Verification items for the finished model (mm, model axes). A direction names the side the tool comes from. Round coordinates to 2 decimals unless told otherwise and drop trailing zeros. Order: outer loops, then holes, each group sorted by start corner. A loop starts at its lowest first (then second) coordinate and runs counter-clockwise, first axis right, second up. Notation, with made-up numbers: (53, 17.5) -> (58, 17.5) arc R6 ccw to (58, 22.5) -> close; hole circle Ø2 at (57, 83.25). An arc over 180 degrees is marked (long way). Return JSON: item names as keys, results as strings. Group by question number.
1) Draft check along X on faces 1 (the cylindrical face through (75.86, 5.64, 12.11)), 2 (the flat face through (86, 25, 12)), 3 (the cylindrical face through (0.71, 50.39, 4.7)). Enter one of: pulls with the +X half, pulls with the -X half, needs draft (parallel to the pull), parting line crosses it, or undercut.
2) Tool access check on faces 4 (the flat face through (2.5, 26, 12)), 5 (the cylindrical face through (83.04, 38.95, 13.05)), 6 (the flat face through (4, 0.4, 4)). Record the directions out of +Z, -Z, +X, -X, +Y, -Y that give a thin tool (end or side, any length) a straight path to the whole face; none if there is none.
3) Section check A-A on x = 30. Enter the section's corners in (y, z).
4) Section check B-B on y = 40.6. Enter the section's corners in (x, z), plus the area to 3 significant figures.
5) Section check C-C on z = 10.5. Enter the section's corners in (x, y).
6) Section check D-D on x = 77.25. Enter the section's corners in (y, z).
7) Depth check by flat-ended pin: pin 1 (2.5 mm diameter, centred on x = 77.25, z = 13, fed in from +Y); pin 2 (1 mm diameter, centred on x = 77.5, z = 12.5, fed in from -Y); pin 3 (6 mm diameter, centred on x = 56, z = 13.5, fed in from -Y). Enter the tip coordinate at first touch or a pass-through.
8) Scan lines: L1, parallel to X at y = 5.8, z = 13; L2, parallel to Z at x = 11, y = 4; L3, parallel to X at y = 21, z = 15.75. Record each from-to range of solid material in increasing order.
Autodesk Fusion 360 part; units mm, degrees
sketch "base" plane through (0, 0, 0) normal (0, 0, 1) x (1, 0, 0)
  line L0 (0, 0) -> (88.5, 0)
  line L1 (88.5, 0) -> (88.5, 48.643)
  line L2 (86, 51.143) -> (2.5, 51.143)
  line L3 (0, 48.643) -> (0, 0)
  arc A0 (2.5, 51.143) -> (0, 48.643) centre (2.5, 48.643) ccw
  arc A1 (88.5, 48.643) -> (86, 51.143) centre (86, 48.643) ccw
  point P0 (0, 51.143)
  dimension "d1" = 88.5
  dimension "d2" = 51.143
  dimension "d14" = 2.5
  dimension "d15" = 2.5
extrude "Extrude1" add sketch "base" along normal blind 8
sketch "inside part" plane through (0, 0, 8) normal (0, 0, 1) x (-1, 0, 0)
  line L0 (0, -48.643) -> (0, 0)
  line L1 (0, 0) -> (-88.5, 0)
  line L2 (-88.5, 0) -> (-88.5, -48.643)
  line L3 (-86, -51.143) -> (-2.5, -51.143)
  line L4 (-2.5, 0) -> (-86, 0)
  line L5 (-86, 0) -> (-86, -48.381)
  line L6 (-85.238, -49.143) -> (-3.262, -49.143)
  line L7 (-2.5, -48.381) -> (-2.5, 0)
  arc A0 (-3.262, -49.143) -> (-2.5, -48.381) centre (-3.262, -48.381) ccw
  arc A1 (-86, -48.381) -> (-85.238, -49.143) centre (-85.238, -48.381) ccw
  arc A2 (-88.5, -48.643) -> (-86, -51.143) centre (-86, -48.643) ccw
  arc A3 (-2.5, -51.143) -> (0, -48.643) centre (-2.5, -48.643) ccw
  dimension "d7" = 2.5
  dimension "d8" = 2.5
  dimension "d9" = 2
  dimension "d12" = 0.762
  dimension "d13" = 0.762
extrude "Extrude2" add sketch "inside part" along normal blind 8 contours L1 L4 L5 L6 L7 A0 A1
fillet "Fillet1" radius 1.5 5 edges at (88.5, 24.3215, 0) (87.7678, 50.4108, 0) (44.25, 51.143, 0) (0.7322, 50.4108, 0) (0, 24.3215, 0)
sketch "Sketch3" plane through (0, 0, 0) normal (0, -1, 0) x (1, 0, 0)
  arc A0 (87, 0) -> (88.5, 1.5) centre (87, 1.5) ccw
  line L0 (88.5, 1.5) -> (88.5, 8)
  line L1 (88.5, 8) -> (86, 8)
  line L2 (86, 8) -> (86, 16)
  line L3 (86, 16) -> (2.5, 16)
  line L4 (2.5, 16) -> (2.5, 8)
  line L5 (2.5, 8) -> (0, 8)
  line L6 (0, 8) -> (0, 1.5)
  arc A1 (0, 1.5) -> (1.5, 0) centre (1.5, 1.5) ccw
  line L7 (1.5, 0) -> (87, 0)
  line L8 (86, 8) -> (2.5, 8)
  line L9 (2.5, 8) -> (2.5, 16)
  line L10 (2.5, 16) -> (86, 16)
  line L11 (86, 16) -> (86, 8)
extrude "Extrude3" cut sketch "Sketch3" against normal blind 2.6 contours L2 L3 L4 L8 L9 L10 L11
sketch "Bottom holes for M2.5 screws" plane through (0, 2.6, 0) normal (0, -1, 0) x (1, 0, 0)
  line L0 (86, 16) -> (2.5, 16)
  line L1 (2.5, 16) -> (2.5, 8)
  line L2 (2.5, 8) -> (86, 8)
  line L3 (86, 8) -> (86, 16)
  line L4 (44.25, 8) -> (44.25, 16) construction
  point P0 (77.25, 13)
  point P1 (11.25, 13)
  dimension "d21" = 33
  dimension "d22" = 33
  dimension "d44" = 5
hole "Hole1" at (11.25, 2.6, 13) at (77.25, 2.6, 13) direction (0, 1, 0) diameter 3.3 depth 6 tip angle 180
sketch "Front/back holes" plane through (86, 0, 0) normal (1, 0, 0) x (0, 1, 0)
  line L0 (2.6, 16) -> (2.6, 8)
  line L1 (2.6, 8) -> (48.381, 8)
  line L2 (48.381, 8) -> (48.381, 16)
  line L3 (48.381, 16) -> (2.6, 16)
  circle A0 centre (8.6, 13) radius 1.65
  circle A1 centre (40.6, 13) radius 1.65
  line L4 (11, 13) -> (9.7344, 14.1982)
  line L5 (11, 13) -> (9.7344, 11.8018)
  line L6 (43, 13) -> (41.7344, 14.1982)
  line L7 (43, 13) -> (41.7344, 11.8018)
  point P0 (8.6, 13)
  point P1 (40.6, 13)
  dimension "d27" = 6
  dimension "d28" = 32
  dimension "d29" = 5
  dimension "d50" = 3.3
  dimension "d51" = 3.3
  dimension "d54" = 2.4
  dimension "d55" = 2.4
extrude "Extrude5" cut sketch "Front/back holes" against normal blind 6 contours A0 | A0 L4 L5 | A1 | A1 L6 L7
sketch "Front/back holes (1)" plane through (2.5, 0, 0) normal (-1, 0, 0) x (0, -1, 0)
  line L0 (-2.6, 8) -> (-2.6, 16)
  line L1 (-2.6, 16) -> (-48.381, 16)
  line L2 (-48.381, 16) -> (-48.381, 8)
  line L3 (-48.381, 8) -> (-2.6, 8)
  circle A0 centre (-40.6, 13) radius 1.65
  circle A1 centre (-8.6, 13) radius 1.65
  line L4 (-43, 13) -> (-41.7344, 11.8018)
  line L5 (-43, 13) -> (-41.7344, 14.1982)
  line L6 (-10.9921, 13) -> (-9.7381, 14.1947)
  line L7 (-10.9921, 13) -> (-9.7381, 11.8053)
  point P0 (-40.6, 13)
  point P1 (-8.6, 13)
  point P2 (-40.6, 13)
  point P3 (-40.6, 13)
  point P4 (-43, 13)
  point P5 (-8.6, 13)
  point P6 (-8.6, 13)
  point P7 (-11, 13)
  dimension "d33" = 6
  dimension "d34" = 32
  dimension "d45" = 5
  dimension "d46" = 3.3
  dimension "d47" = 3.3
  dimension "d56" = 2.4
  dimension "d57" = 2.4
extrude "Extrude4" cut sketch "Front/back holes (1)" against normal blind 6 contours A0 | A0 L4 L5 | A1 | A1 L6 L7
sketch "Sketch8" plane through (0, 0, 0) normal (0, -1, 0) x (1, 0, 0)
  line L0 (88.5, 8) -> (0, 8)
  line L1 (0, 8) -> (0, 1.5)
  arc A0 (0, 1.5) -> (1.5, 0) centre (1.5, 1.5) ccw
  line L2 (1.5, 0) -> (87, 0)
  arc A1 (87, 0) -> (88.5, 1.5) centre (87, 1.5) ccw
  line L3 (88.5, 1.5) -> (88.5, 8)
  line L4 (88.5, 4) -> (0, 4) construction
  point P0 (4, 4)
  point P1 (84.5, 4)
  dimension "d58" = 4
  dimension "d59" = 4
  dimension "d60" = 4
  dimension "d61" = 4
hole "Hole4" at (4, 0, 4) at (84.5, 0, 4) direction (0, 1, 0) diameter 6.1 depth 0.4 tip angle 180
equation "d1 = 83.5 mm + 2 * extrawidth"
equation "d2 = extraheight + 49.143 mm"
equation "extrawidth = 2.5 mm"
equation "extraheight = 2 mm"
equation "d7 = extrawidth"
equation "d8 = extrawidth"
equation "d9 = extraheight"
Check result:
{
 "1": {"face 1": "undercut", "face 2": "pulls with the +X half", "face 3": "pulls with the -X half"},
 "2": {"face 4": "+Z, -X, +Y, -Y", "face 5": "+X", "face 6": "-Y"},
 "3": {"outline": "(0, 0) -> (49.64, 0) arc R1.5 ccw to (51.14, 1.5) -> (51.14, 8) -> (49.14, 8) -> (49.14, 16) -> (2.6, 16) -> (2.6, 8) -> (0, 8) -> close"},
 "4": {"outline": "(0, 1.5) arc R1.5 ccw to (1.5, 0) -> (87, 0) arc R1.5 ccw to (88.5, 1.5) -> (88.5, 8) -> (86, 8) -> (86, 11.35) -> (80, 11.35) -> (80, 14.65) -> (86, 14.65) -> (86, 16) -> (2.5, 16) -> (2.5, 14.65) -> (8.5, 14.65) -> (8.5, 11.35) -> (2.5, 11.35) -> (2.5, 8) -> (0, 8) -> close", "area": "1,340 mm^2"},
 "5": {"outline": "(2.5, 2.6) -> (86, 2.6) -> (86, 48.38) arc R0.76 ccw to (85.24, 49.14) -> (3.26, 49.14) arc R0.76 ccw to (2.5, 48.38) -> close"},
 "6": {"outline": "(0, 0) -> (49.64, 0) arc R1.5 ccw to (51.14, 1.5) -> (51.14, 8) -> (49.14, 8) -> (49.14, 16) -> (2.6, 16) -> (2.6, 14.65) -> (8.6, 14.65) -> (8.6, 11.35) -> (2.6, 11.35) -> (2.6, 8) -> (0, 8) -> close"},
 "7": {"pin 1": "y = 49.14", "pin 2": "y = 8.6", "pin 3": "y = 2.6"},
 "8": {"L1": "2.5 to 9.6, 12.9 to 75.6, 78.9 to 86", "L2": "0 to 11.37, 14.63 to 16", "L3": "2.5 to 86"}
}
